```python
from build123d import *

# Parameters (mm, degrees)
BOSS_EXTRUDE1_DEPTH = 76.2
SKETCH6_R           = 7.5
CUT_EXTRUDE1_DEPTH  = 164


with BuildPart() as part:
    # Sketch1 → Boss-Extrude1 (new body)
    with BuildSketch(Plane(origin=(0, 0, 0), x_dir=(1, 0, 0), z_dir=(0, 1, 0))):
        with BuildLine():
            ThreePointArc((-630.001110861, -32.499999959), (-658.488874236, 15.640781416), (-602.579780619, 17.446534545))
            Line((-602.579780619, 17.446534545), (-589.924302497, 25.498776329))
            ThreePointArc((-589.924302497, 25.498776329), (-671.63274562, 22.868397775), (-630.021699517, -47.499985829))
            ThreePointArc((-630.021699517, -47.499985829), (0, -163), (630.021699517, -47.499985829))
            ThreePointArc((630.021699517, -47.499985829), (671.63274562, 22.868397775), (589.924302497, 25.498776329))
            Line((589.924302497, 25.498776329), (602.579780619, 17.446534545))
            ThreePointArc((602.579780619, 17.446534545), (658.488874236, 15.640781416), (630.001110861, -32.499999959))
            ThreePointArc((630.001110861, -32.499999959), (0, -148), (-630.001110861, -32.499999959))
        make_face()
    extrude(amount=BOSS_EXTRUDE1_DEPTH)

    # Sketch6 → Cut-Extrude1 (cut, through all)
    with BuildSketch(Plane.XY):
        with Locations((0, 38.1)):
            Circle(SKETCH6_R)
    extrude(amount=CUT_EXTRUDE1_DEPTH, mode=Mode.SUBTRACT)


solid = part.part
```
Model file for the job. Use its own axes, mm. Coordinates: 2 decimals unless noted, no trailing zeros. Order: outer loops, then holes, each group sorted by start corner. A loop starts at its lowest first (then second) coordinate and runs counter-clockwise, first axis right, second up. Notation, with made-up numbers: (69.5, 75) -> (84.5, 75) arc R24 ccw to (84.5, 107) -> close; hole circle Ø10 at (14.5, 27). An arc over 180 degrees is marked (long way). Answer as a JSON object with one key per item and string values. Group by question number.
1) Cut at D-D, the plane x = -445.5. Write the cut outline in (y, z), then the cut area to 3 significant figures.
2) Drill centre lines: L1, parallel to Y at x = 0, z = 155.75; L2, parallel to X at y = 53, z = 0; L3, parallel to Z at x = -630, y = 29. Where is each one in solid material? Low to high.
3) Cut at C-C, the plane x = 463.5. Write the cut outline in (y, z), then the cut area to 3 significant figures.
4) Flat gauge pins, fed straight in: pin 1 (8 mm diameter, centred on y = 35, z = 26.5, fed in from +X); pin 2 (6 mm diameter, centred on x = 457, y = 38.5, fed in from -Z). Where does each tip first touch, or does it go through?
5) Pull direction X, two halves, no side cores. Call faces 1 (the face through (672.28, 37.57, -21.65)), 2 (the face through (-3, 0, 151)), 3 (the face through (-9.017, 37.567, 162.977)): +X half, -X half, draft (parallel to the pull), parting line (faces both ways), or undercut.
Check values:
{
 "1": {"outline": "(0, 91.21) -> (76.2, 91.21) -> (76.2, 106.22) -> (0, 106.22) -> close", "area": "1,140 mm²"},
 "2": {"L1": "y = 0 to 30.6, 45.6 to 76.2", "L2": "x = -677.5 to -662.5, 662.5 to 677.5", "L3": "z = -47.5 to -32.5, 32.5 to 47.51"},
 "3": {"outline": "(0, 86.45) -> (76.2, 86.45) -> (76.2, 101.45) -> (0, 101.45) -> close", "area": "1,140 mm²"},
 "4": {"pin 1": "stops at x = 671.83", "pin 2": "stops at z = 87.39"},
 "5": {"face 1": "undercut", "face 2": "draft", "face 3": "parting line"}
}
